Autodesk Inventor part; units mm, degrees
ref_plane "YZ Plane" through (0, 0, 0) normal (1, 0, 0) x (0, 1, 0)
ref_plane "XZ Plane" through (0, 0, 0) normal (0, 1, 0) x (-1, 0, 0)
ref_plane "XY Plane" through (0, 0, 0) normal (0, 0, 1) x (1, 0, 0)
sketch "Sketch1" plane through (0, 0, 0) normal (0, 0, 1) x (1, 0, 0)
  line L0 (-120, 15) -> (120, 15)
  line L1 (120, -15) -> (-120, -15)
  line L2 (-120, 15) -> (120, -15) construction
  line L3 (120, 15) -> (-120, -15) construction
  arc A0 (-107.7136, -0.75) -> (-107.7136, 0.75) centre (-100, 0) ccw
  line L4 (0, -11.513) -> (0, 11.513)
  line L5 (-107.7136, 0.75) -> (-120, 0.75)
  line L6 (-107.7136, -0.75) -> (-120, -0.75)
  line L7 (-120, -15) -> (-120, -0.75)
  line L8 (-120, 0.75) -> (-120, 15)
  arc A1 (107.7136, 0.75) -> (107.7136, -0.75) centre (100, 0) ccw
  line L9 (107.7136, 0.75) -> (120, 0.75)
  line L10 (107.7136, -0.75) -> (120, -0.75)
  line L11 (120, 15) -> (120, 0.75)
  line L12 (120, -0.75) -> (120, -15)
  circle A2 centre (0, 0) radius 5.5
  circle A3 centre (0, 8) radius 2
  circle A4 centre (8, 0) radius 2
  circle A5 centre (0, -8) radius 2
  circle A6 centre (-8, 0) radius 2
  dimension "d0" = 240
  dimension "d1" = 30
  dimension "d3" = 15.5
  dimension "d6" = 100
  dimension "d7" = 11
  dimension "d9" = 4
  dimension "d10" = 4
  dimension "d11" = 4
  dimension "d12" = 4
extrude "Extrusion1" add sketch "Sketch1" along normal blind 25
sketch "Sketch2" plane through (-120, -15, 0) normal (0, -1, 0) x (1, 0, 0)
  line L0 (120, 0) -> (120, 25)
  line L1 (12.2864, 0) -> (12.2864, 25)
  line L2 (0, 25) -> (240, 25)
  line L3 (12.2864, 0) -> (64.2864, 0)
  line L4 (64.2864, 0) -> (64.2864, 25)
  line L5 (12.2864, 25) -> (12.2864, 0)
  line L6 (59.2864, 25) -> (59.2864, 5)
  line L7 (59.2864, 5) -> (17.2864, 5)
  line L8 (17.2864, 5) -> (17.2864, 25)
  line L9 (64.2864, 25) -> (59.2864, 25)
  line L10 (17.2864, 25) -> (12.2864, 25)
  line L11 (227.7136, 0) -> (227.7136, 25)
  line L12 (240, 25) -> (0, 25)
  line L13 (227.7136, 0) -> (175.7136, 0)
  line L14 (175.7136, 0) -> (175.7136, 25)
  line L15 (227.7136, 25) -> (227.7136, 0)
  line L16 (180.7136, 25) -> (180.7136, 5)
  line L17 (180.7136, 5) -> (222.7136, 5)
  line L18 (222.7136, 5) -> (222.7136, 25)
  line L19 (175.7136, 25) -> (180.7136, 25)
  line L20 (222.7136, 25) -> (227.7136, 25)
  line L21 (240, 0) -> (0, 0)
  dimension "d23" = 52
  dimension "d24" = 5
  dimension "d28" = 0
  dimension "d30" = 20
sketch "Sketch3" plane through (120, -15, 0) normal (0, -1, 0) x (1, 0, 0)
  point P0 (-120, 0)
extrude "Extrusion4" add sketch "Sketch2" along normal blind 25 contours L14 L2 L16 L17 L18 L11 L13 | L3 L1 L2 L8 L7 L6 L4
sketch "Sketch4" plane through (120, -15, 0) normal (0, -1, 0) x (1, 0, 0)
  line L0 (-240, 0) -> (0, 0)
  line L1 (-12.2864, 25) -> (0, 25)
  circle A0 centre (-6.1432, 12.5) radius 2.75
  line L2 (-120, 0) -> (-120, 25)
  line L3 (-122, 0) -> (-122, 25)
  circle A1 centre (-233.8568, 12.5) radius 2.75
  dimension "d33" = 5.5
hole "Hole1" at (113.8568, -15, 12.5) at (-113.8568, -15, 12.5) direction (0, 1, 0) diameter 5.5 end through all
sketch "Sketch5" plane through (-107.7136, -15, 0) normal (-1, 0, 0) x (0, 0, 1)
  line L0 (5, 0) -> (5, -25)
  line L1 (5, 0) -> (24.9936, -25)
  circle A0 centre (14.9968, -12.5) radius 2.75
  point P0 (0, 15)
  dimension "d41" = 5.5
extrude "Extrusion5" cut sketch "Sketch5" against normal through all
chamfer "Chamfer2" distance 5 angle 45 2 edges at (-55.7136, -15, 12.5) (55.7136, -15, 12.5)
chamfer "Chamfer3" distance 2 angle 45 2 edges at (-107.7136, -15, 12.5) (107.7136, -15, 12.5)
fillet "Fillet2" radius 2 8 edges at (120, -15, 12.5) (120, 15, 12.5) (105.2136, -40, 25) (58.2136, -40, 25) (-58.2136, -40, 25) (-105.2136, -40, 25) (-120, -15, 12.5) (-120, 15, 12.5)
properties part number "Trava Z"
Model file for the job. Use its own axes, mm. A direction names the side the tool comes from. Give positions to 0.01 mm unless a question says otherwise; leave off trailing zeros. Loops run counter-clockwise (first coordinate to the right, second up) from the corner with the lowest first, then second, coordinate; pieces in that order, holes last.
Item 1: Drop flat-ended pins along their axis: P1, Ø6, axis at x = 84.5, z = 19, coming from the -Y side; P2, Ø3, axis at y = -18, z = 21.5, coming from the +X side; P3, Ø6, axis at y = -23.5, z = 11, coming from the -X side. Give the stop position or say it passes through.
Check values:
P1: stops at y = -15
P2: stops at x = 108.21
P3: stops at x = -107.71
Item 2: Slice it at A-A (y = -27.5). Give the number of separate pieces and of enclosed holes in the cut face, plus the area to 3 significant figures.
Check values:
separate pieces: 6
enclosed holes: 0
area: 810 mm2
Item 3: Slice it at B-B (x = -100). Write the cut outline in (y, z).
Check values:
outline: (-40, 0) - (-7.75, 0) - (-7.75, 25) - (-15, 25) - (-15, 5) - (-40, 5) - close; (7.75, 0) - (15, 0) - (15, 25) - (7.75, 25) - close
Item 4: Which spindle directions (+Z, -Z, +X, -X, +Y, -Y) get a long thin tool onto all of the face, cutting with end or side? Do faces 3 (the face through (-113.8, -15, 9.5)), 4 (the face through (102.714, -24.5, 14.9)), 5 (the face through (-55.714, -30, 12)), 6 (the face through (-9.6, 1.2, 12.3)). Say none if no direction does.
Check values:
face 3: +Z, -Z, -X, -Y
face 4: +Z, -Y
face 5: +Z, -Z, -Y
face 6: +Z, -Z
Item 5: Mould opens along Z. For faces 1 (the face through (105.18, -26.67, 17.62)), 2 (the face through (-107.714, -28, 12)) say: +Z half, -Z half, draft (parallel to the pull), parting line (faces both ways), or undercut.
Check values:
face 1: undercut
face 2: draft
Item 6: Drill centre lines: line 1 along X through (y, z) = (-8, 12); line 2 along X through (y, z) = (-8, 17.5); line 3 along X through (y, z) = (-36.5, 20.75). Where is each one in solid material? Low to high.
Check values:
line 1: x = -120 to -116.56, -111.15 to -2, 2 to 111.15, 116.56 to 120
line 2: x = -120 to -2, 2 to 120
line 3: x = -107.71 to -102.71, -60.71 to -55.71, 55.71 to 60.71, 102.71 to 107.71
Item 7: Slice it at C-C (x = 8). Write the cut outline in (y, z).
Check values:
outline: (-15, 0) - (-2, 0) - (-2, 25) - (-15, 25) - close; (2, 0) - (15, 0) - (15, 25) - (2, 25) - close
